Here's how the part is built. I have some questions about the finished solid (model axes, mm). A direction names the side the tool comes from. Coordinates: 2 decimals unless noted, no trailing zeros. Loops run counter-clockwise (first coordinate to the right, second up) from the corner with the lowest first, then second, coordinate; pieces in that order, holes last. Notation, with made-up numbers: M -37,20 L -24,20 A5 cw -24,25 Z; hole C 78.5,-32.75 d10. An arc over 180 degrees is marked long. Use one line per item in the form item = value. Start each with the question number.
(1) Imagine slicing it at A-A, the plane y = 0. Please give me the cut outline in (x, z).
(2) Will these pins go through, and if not, where does the flat tip stop? P1, Ø3, axis at y = -1, z = 19, coming from the +X side; P2, Ø1, axis at y = -5, z = 13, coming from the -X side; P3, Ø1.5, axis at y = 7.5, z = 4, coming from the +X side.
(3) Please list where these lines run through material, in increasing order: L1, parallel to Y at x = 0, z = 14.5; L2, parallel to X at y = 0, z = 21.25; L3, parallel to Y at x = -1, z = 28.
(4) Imagine slicing it at B-B, the plane z = 25.5. Please give me the cut outline in (x, y).
(5) On a 3-axis mill with a long thin cutter (end or side, diameter ignored), from which of +Z, -Z, +X, -X, +Y, -Y can I reach the whole of each face in a straight line? I mean faces 1 (the cylindrical face through (-9.8, -2.22, 14.12)), 2 (the cylindrical face through (-4.25, 8.94, 14.12)), 3 (the cylindrical face through (4.35, -9.06, 14.12)), 4 (the cylindrical face through (-2.059, 9.274, 27.236)). Say none if no direction works.
(6) Thinking about a two-plate mould opening in Y: for faces 5 (the cylindrical face through (-3.354, 0.676, 14.79)), 6 (the cylindrical face through (0, -9.9, 14.1)), 7 (the conical face through (0.01, 8.7, 29.35)), which applies, +Y half, -Y half, draft (parallel to the pull), parting line (faces both ways), or undercut?
```python
from build123d import *

# Parameters (mm, degrees)
AUFSATZ_LINEAR_AUSTRAGEN1_DEPTH      = 30
SKIZZE2_R                            = 11
AUFSATZ_LINEAR_AUSTRAGEN2_DEPTH      = 2
FASE1_SIZE                           = 2
SCHNITT_LINEAR_AUSTRAGEN1_DEPTH      = 33.031234844
SCHNITT_LINEAR_AUSTRAGEN1_DEPTH_BACK = 33.031234844
SKIZZE3_R                            = 2.25


with BuildPart() as part:
    # Skizze1 → Aufsatz-Linear austragen1 (new body)
    with BuildSketch(Plane.XY):
        with BuildLine():
            ThreePointArc((9.834694469, -1.13524654), (9.651786331, 2.202957246), (8.368188528, 5.289935799))
            ThreePointArc((8.368188528, 5.289935799), (7.857406399, 6.266072509), (7.019403191, 6.981259116))
            ThreePointArc((7.019403191, 6.981259116), (4.295449017, 8.919591792), (1.081641859, 9.840734266))
            ThreePointArc((1.081641859, 9.840734266), (0, 10.05), (-1.081641859, 9.840734266))
            ThreePointArc((-1.081641859, 9.840734266), (-4.295449017, 8.919591792), (-7.019403191, 6.981259116))
            ThreePointArc((-7.019403191, 6.981259116), (-7.857406399, 6.266072509), (-8.368188528, 5.289935799))
            ThreePointArc((-8.368188528, 5.289935799), (-9.651786331, 2.202957246), (-9.834694469, -1.13524654))
            ThreePointArc((-9.834694469, -1.13524654), (-9.798025517, -2.236335386), (-9.353318555, -3.244292219))
            ThreePointArc((-9.353318555, -3.244292219), (-7.740131676, -6.172549038), (-5.24426022, -8.396888397))
            ThreePointArc((-5.24426022, -8.396888397), (-4.360531578, -9.054737122), (-3.295208938, -9.335502025))
            ThreePointArc((-3.295208938, -9.335502025), (0, -9.9), (3.295208938, -9.335502025))
            ThreePointArc((3.295208938, -9.335502025), (4.360531578, -9.054737122), (5.24426022, -8.396888397))
            ThreePointArc((5.24426022, -8.396888397), (7.740131676, -6.172549038), (9.353318555, -3.244292219))
            ThreePointArc((9.353318555, -3.244292219), (9.798025517, -2.236335386), (9.834694469, -1.13524654))
        make_face()
    extrude(amount=AUFSATZ_LINEAR_AUSTRAGEN1_DEPTH)

    # Skizze2 → Aufsatz-Linear austragen2 (add)
    with BuildSketch(Plane.XY):
        Circle(SKIZZE2_R)
    extrude(amount=AUFSATZ_LINEAR_AUSTRAGEN2_DEPTH)

    # Fase1
    fase1_edges = [part.edges().sort_by_distance(p)[0] for p in [
        (7.857406399, 6.266072509, 30),
        (4.295449017, 8.919591792, 30),
        (0, 10.05, 30),
        (-4.295449017, 8.919591792, 30),
        (-7.857406399, 6.266072509, 30),
        (-9.651786331, 2.202957246, 30),
        (-9.798025517, -2.236335386, 30),
        (-7.740131676, -6.172549038, 30),
        (-4.360531578, -9.054737122, 30),
        (0, -9.9, 30),
        (9.651786331, 2.202957246, 30),
        (4.360531578, -9.054737122, 30),
        (7.740131676, -6.172549038, 30),
        (9.798025517, -2.236335386, 30),
    ]]
    chamfer(fase1_edges, length=FASE1_SIZE)

    # Skizze3 → Schnitt-Linear austragen1 (cut, two sides: drawn at the far end of the back side and taken through both)
    with BuildSketch(Plane.XY.offset(2).offset(-SCHNITT_LINEAR_AUSTRAGEN1_DEPTH_BACK)):
        with Locations((0, 5.5)):
            Circle(SKIZZE3_R)
        with Locations((5.5, 0)):
            Circle(SKIZZE3_R)
        with Locations((0, -5.5)):
            Circle(SKIZZE3_R)
        with Locations((-5.5, 0)):
            Circle(SKIZZE3_R)
    extrude(amount=SCHNITT_LINEAR_AUSTRAGEN1_DEPTH + SCHNITT_LINEAR_AUSTRAGEN1_DEPTH_BACK, mode=Mode.SUBTRACT)

    # Skizze4 → Schnitt-Rotation1 (revolve, cut)
    with BuildSketch(Plane(origin=(0, 0, 0), x_dir=(0, 0, -1), z_dir=(1, 0, 0)), mode=Mode.PRIVATE) as schnitt_rotation1_sk:
        Polygon((-27.876581368, 10.05), (-26.576581368, 10.05), (-26.576581368, 9.5), (-27.876581368, 9.5), (-29.929209312, 10.05), align=None)
    revolve(schnitt_rotation1_sk.sketch.rotate(Axis((0, 0, 0), (0, 0, -1)), 90), axis=Axis((0, 0, 0), (0, 0, -1)), mode=Mode.SUBTRACT)


solid = part.part
```
Answer:
q1.outline = M -11,0 L -7.75,0 L -7.75,30 L -7.9,30 L -9.61,28.29 L -9.5,27.88 L -9.5,26.58 L -9.9,26.58 L -9.9,2 L -11,2 Z; M -3.25,0 L 3.25,0 L 3.25,30 L -3.25,30 Z; M 7.75,0 L 11,0 L 11,2 L 9.9,2 L 9.9,26.58 L 9.5,26.58 L 9.5,27.88 L 9.61,28.29 L 7.9,30 L 7.75,30 Z
q2.P1 = 9.9
q2.P2 = -8.82
q2.P3 = 7.37
q3.L1 = -9.9 to -7.75, -3.25 to 3.25, 7.75 to 10.05
q3.L2 = -9.9 to -7.75, -3.25 to 3.25, 7.75 to 9.9
q3.L3 = -9.48 to -7.52, -3.48 to 3.48, 7.52 to 9.48
q4.outline = M -9.83,-1.14 A2.9 ccw -9.35,-3.24 A9.9 ccw -5.24,-8.4 A2.9 ccw -3.3,-9.34 A9.9 ccw 3.3,-9.34 A2.9 ccw 5.24,-8.4 A9.9 ccw 9.35,-3.24 A2.9 ccw 9.83,-1.14 A9.9 ccw 8.37,5.29 A2.9 ccw 7.02,6.98 A9.9 ccw 1.08,9.84 A2.9 ccw -1.08,9.84 A9.9 ccw -7.02,6.98 A2.9 ccw -8.37,5.29 A9.9 ccw Z; hole C -5.5,0 d4.5; hole C 0,-5.5 d4.5; hole C 0,5.5 d4.5; hole C 5.5,0 d4.5
q5.face_1 = +Z, -X
q5.face_2 = +Z, -X, +Y
q5.face_3 = +Z, +X, -Y
q5.face_4 = none
q6.face_5 = undercut
q6.face_6 = -Y half
q6.face_7 = +Y half
